Input: part model. Units: mm. Frame: model coordinates. Give positions to 0.01 mm unless a question says otherwise; leave off trailing zeros. Loops run counter-clockwise (first coordinate to the right, second up) from the corner with the lowest first, then second, coordinate; pieces in that order, holes last. Notation, with made-up numbers: (89, 54.5) - (136, 54.5) arc R18 ccw to (136, 78.5) - close; hole circle Ø5 at (26, -9). An arc over 180 degrees is marked (long way). Answer as a JSON object with one key per item and string values. Group by question number.
(1) Section query D-D (z = 2). Count the separate pieces of the cut face and the enclosed holes in it, plus the area to 3 significant figures.
(2) Section query A-A (y = 74). Return loops of the section in (x, z), plus the area to 3 significant figures.
(3) Section query C-C (x = 185.5). Return loops of the section in (y, z), plus the area to 3 significant figures.
(4) Section query B-B (x = 209). Return loops of the section in (y, z).
(5) Material intervals for L1, parallel to Y at x = 147.5, z = 2.6; L2, parallel to Y at x = 245, z = 2.75; L3, parallel to X at y = 65.5, z = 0.7, sorted ascending.
(6) Pin query (flat end, axial travel): P1, Ø1.5, axis at x = 148.5, z = 1.5, coming from the -Y side; P2, Ø3.5, axis at x = 174, y = 13.71, coming from the -Z side; P3, Ø0.9, axis at x = 150.5, z = 2, coming from the +Y side; P4, Ø0.9, axis at y = 72.5, z = 1, coming from the -X side. Return the tip coordinate at first contact, or that it passes through.
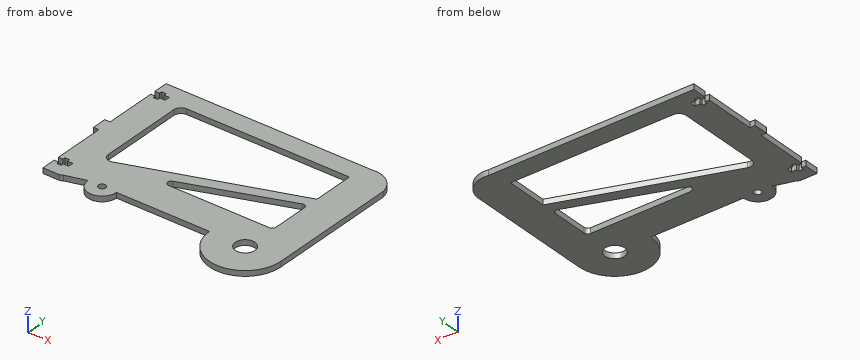
```python
from build123d import *

# Parameters (mm, degrees)
SKETCH_1_R      = 2
SKETCH_1_R_2    = 5.5
EXTRUDE_1_DEPTH = 3


with BuildPart() as part:
    # 草图1 → 凸台-拉伸1 (new body)
    with BuildSketch(Plane.XY):
        with BuildLine():
            Line((234.002581869, 13.707860978), (182.002581869, 13.707860978))
            ThreePointArc((182.002581869, 13.707860978), (174.002581869, 5.707860978), (166.002581869, 13.707860978))
            Line((166.002581869, 13.707860978), (154.850930387, 10.484571811))
            ThreePointArc((154.850930387, 10.484571811), (153.916116795, 9.908765811), (152.836734449, 9.707860978))
            Line((152.836734449, 9.707860978), (144.002581869, 9.707860978))
            Line((144.002581869, 9.707860978), (144.002581869, 17.707860978))
            Line((144.002581869, 17.707860978), (146.502581869, 17.707860978))
            Line((146.502581869, 17.707860978), (146.502581869, 16.207860978))
            Line((146.502581869, 16.207860978), (149.102581869, 16.207860978))
            Line((149.102581869, 16.207860978), (149.102581869, 17.707860978))
            Line((149.102581869, 17.707860978), (152.102581869, 17.707860978))
            Line((152.102581869, 17.707860978), (152.102581869, 20.707860978))
            Line((152.102581869, 20.707860978), (149.102581869, 20.707860978))
            Line((149.102581869, 20.707860978), (149.102581869, 22.207860978))
            Line((149.102581869, 22.207860978), (146.502581869, 22.207860978))
            Line((146.502581869, 22.207860978), (146.502581869, 20.707860978))
            Line((146.502581869, 20.707860978), (144.002581869, 20.707860978))
            Line((144.002581869, 20.707860978), (144.002581869, 49.707860978))
            Line((144.002581869, 49.707860978), (141.002581869, 49.707860978))
            Line((141.002581869, 49.707860978), (141.002581869, 57.707860978))
            Line((141.002581869, 57.707860978), (144.002581869, 57.707860978))
            Line((144.002581869, 57.707860978), (144.002581869, 86.707860978))
            Line((144.002581869, 86.707860978), (146.502581869, 86.707860978))
            Line((146.502581869, 86.707860978), (146.502581869, 85.207860978))
            Line((146.502581869, 85.207860978), (149.102581869, 85.207860978))
            Line((149.102581869, 85.207860978), (149.102581869, 86.707860978))
            Line((149.102581869, 86.707860978), (152.102581869, 86.707860978))
            Line((152.102581869, 86.707860978), (152.102581869, 89.707860978))
            Line((152.102581869, 89.707860978), (149.102581869, 89.707860978))
            Line((149.102581869, 89.707860978), (149.102581869, 91.207860978))
            Line((149.102581869, 91.207860978), (146.502581869, 91.207860978))
            Line((146.502581869, 91.207860978), (146.502581869, 89.707860978))
            Line((146.502581869, 89.707860978), (144.002581869, 89.707860978))
            Line((144.002581869, 89.707860978), (144.002581869, 97.707860978))
            Line((144.002581869, 97.707860978), (154.002581869, 97.707860978))
            Line((154.002581869, 97.707860978), (259.002581869, 97.707860978))
            ThreePointArc((259.002581869, 97.707860978), (268.727085047, 95.444036955), (274.002581869, 86.967009497))
            Line((274.002581869, 86.967009497), (274.002581869, 13.707860978))
            ThreePointArc((274.002581869, 13.707860978), (254.002581869, -6.292139022), (234.002581869, 13.707860978))
        make_face()
        with Locations((174.002581869, 13.707860978)):
            Circle(SKETCH_1_R, mode=Mode.SUBTRACT)
        with Locations((254.002581869, 13.707860978)):
            Circle(SKETCH_1_R_2, mode=Mode.SUBTRACT)
        with BuildLine():
            Line((165.194921817, 32.396144085), (255.002581869, 63.765533121))
            Line((255.002581869, 63.765533121), (255.002581869, 86.967009497))
            Line((255.002581869, 86.967009497), (163.875891268, 86.967009497))
            ThreePointArc((163.875891268, 86.967009497), (161.047464143, 85.795436622), (159.875891268, 82.967009497))
            Line((159.875891268, 82.967009497), (159.875891268, 36.172406577))
            ThreePointArc((159.875891268, 36.172406577), (161.560305186, 32.910802508), (165.194921817, 32.396144085))
        make_face(mode=Mode.SUBTRACT)
        with BuildLine():
            Line((195.793134982, 36.276744779), (252.321890288, 56.737573029))
            ThreePointArc((252.321890288, 56.737573029), (254.151193387, 56.494254101), (255.002581869, 54.856972335))
            Line((255.002581869, 54.856972335), (255.002581869, 34.396144085))
            ThreePointArc((255.002581869, 34.396144085), (254.416795432, 32.981930522), (253.002581869, 32.396144085))
            Line((253.002581869, 32.396144085), (196.473826563, 32.396144085))
            ThreePointArc((196.473826563, 32.396144085), (194.50390253, 34.050602038), (195.793134982, 36.276744779))
        make_face(mode=Mode.SUBTRACT)
    extrude(amount=EXTRUDE_1_DEPTH)


solid = part.part
```
Recorded:
{
 "1": {"separate pieces": "1", "enclosed holes": "4", "area": "6,890 mm^2"},
 "2": {"outline": "(144, 0) - (159.88, 0) - (159.88, 3) - (144, 3) - close; (255, 0) - (274, 0) - (274, 3) - (255, 3) - close", "area": "105 mm^2"},
 "3": {"outline": "(13.71, 0) - (39.49, 0) - (39.49, 3) - (13.71, 3) - close; (86.97, 0) - (97.71, 0) - (97.71, 3) - (86.97, 3) - close", "area": "110 mm^2"},
 "4": {"outline": "(13.71, 0) - (32.4, 0) - (32.4, 3) - (13.71, 3) - close; (41.06, 0) - (47.7, 0) - (47.7, 3) - (41.06, 3) - close; (86.97, 0) - (97.71, 0) - (97.71, 3) - (86.97, 3) - close"},
 "5": {"L1": "y = 9.71 to 16.21, 22.21 to 85.21, 91.21 to 97.71", "L2": "y = -4.15 to 32.4, 54.09 to 60.27, 86.97 to 97.71", "L3": "x = 144 to 159.88, 255 to 274"},
 "6": {"P1": "stops at y = 9.71", "P2": "passes through", "P3": "stops at y = 97.71", "P4": "stops at x = 144"}
}
